For this review, use the dimensioned drawing (mm, ordinates from the lowest corner) and the shaded views. Coordinates: 2 decimals unless noted, no trailing zeros. Loops run counter-clockwise (first coordinate to the right, second up) from the corner with the lowest first, then second, coordinate; pieces in that order, holes last. Notation, with made-up numbers: M 67,31 L 113,31 A13 cw 113,35 Z; hole C 75.25,-27 d1. An arc over 180 degrees is marked long. Write item = value, one per line.
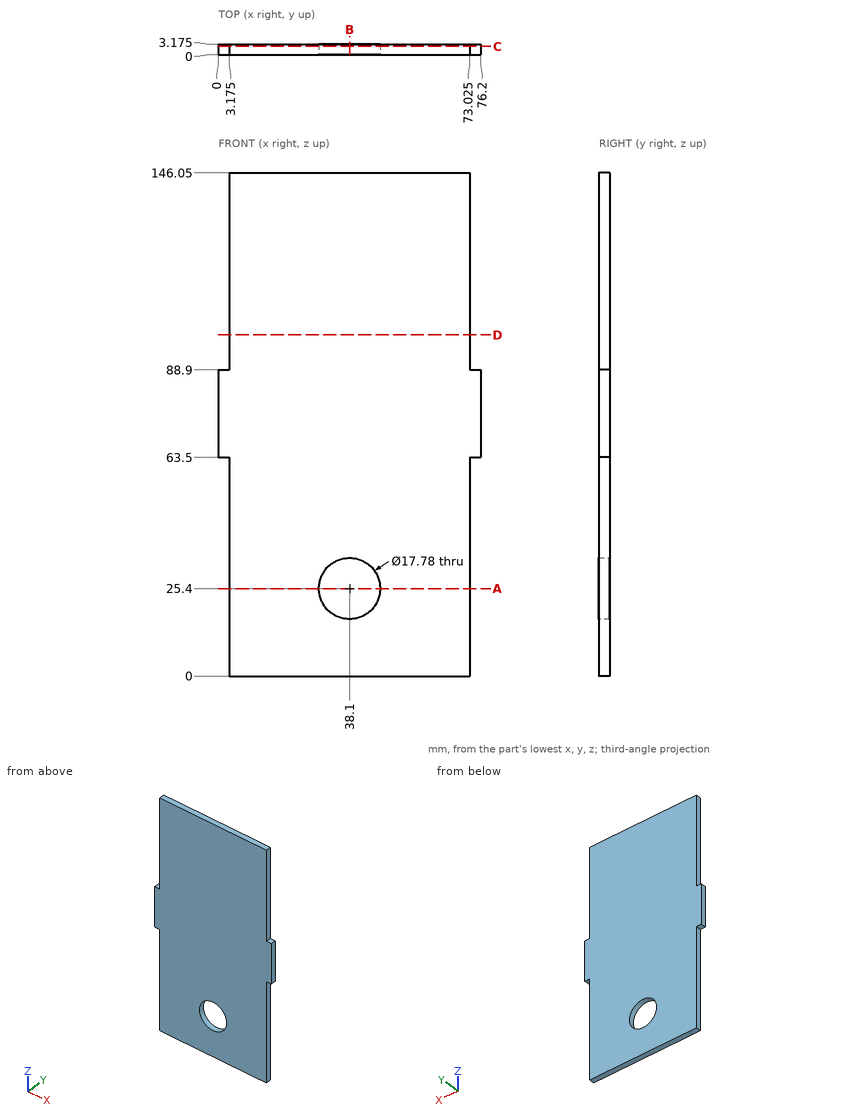
Q1. Add section D-D (z = 99). Write out the cut boundary in (x, y) (3 decimals), and give its area (3 significant figures).
Solved:
outline = M 3.175,0 L 73.025,0 L 73.025,3.175 L 3.175,3.175 Z
area = 222 mm²
Q2. For line 1 along X through (y, z) = (1.95, 25.4) (3 decimals); line 2 along X through (y, z) = (0.65, 53) (3 decimals); line 3 along X through (y, z) = (0.5, 19) (3 decimals), list the stretches that pass through material, from the lowest coordinate up.
Solved:
line_1 = 3.175 to 29.21, 46.99 to 73.025
line_2 = 3.175 to 73.025
line_3 = 3.175 to 31.93, 44.27 to 73.025
Q3. Add section A-A (z = 25.4). Write out the cut boundary in (x, y) (3 decimals).
Solved:
outline = M 3.175,0 L 29.21,0 L 29.21,3.175 L 3.175,3.175 Z; M 46.99,0 L 73.025,0 L 73.025,3.175 L 46.99,3.175 Z
Q4. For pin 1 Ø5 at (x, z) = (29, 34.5) entering from -Y; pin 2 Ø1 at (y, z) = (1.5, 19.5) entering from -X (3 decimals); pin 3 Ø1 at (x, y) = (1.5, 1) entering from -Z; pin 4 Ø16 at (x, z) = (38.1, 25.4) entering from -Y, all flat-tipped, find the tip position at first contact; note any pin that passes through.
Solved:
pin_1 = 0
pin_2 = 3.175
pin_3 = 63.5
pin_4 = through
Q5. Add section C-C (y = 2.5). Write out the cut boundary in (x, z) (3 decimals), and give its area (3 significant figures).
Solved:
outline = M 0,63.5 L 3.175,63.5 L 3.175,0 L 73.025,0 L 73.025,63.5 L 76.2,63.5 L 76.2,88.9 L 73.025,88.9 L 73.025,146.05 L 3.175,146.05 L 3.175,88.9 L 0,88.9 Z; hole C 38.1,25.4 d17.78
area = 10,100 mm²
Q6. Add section B-B (x = 38.1). Write out the cut boundary in (y, z) (3 decimals), and give its area (3 significant figures).
Solved:
outline = M 0,0 L 3.175,0 L 3.175,16.51 L 0,16.51 Z; M 0,34.29 L 3.175,34.29 L 3.175,146.05 L 0,146.05 Z
area = 407 mm²
